```python
from build123d import *

# Parameters (mm, degrees)
F1_DEPTH  = 6
F3_R      = 2.5
F4_DEPTH  = 25
F5_W      = 22.1
F5_H      = 30
F6_DEPTH  = 25
F7_R      = 8
F7_R_2    = 12
F7_R_3    = 1.25
F8_DEPTH  = 25
F9_R      = 1
F10_DEPTH = 3
F11_R     = 1
F12_DEPTH = 3


with BuildPart() as f1:
    # F0 (on Top) → F1 (new body)
    with BuildSketch(Plane.XY):
        Polygon((0, -73.897189), (0, -125), (224, -125), (224, -73.897189), (383.758505, -30), (440.241495, -14.480047), (431.678371, 14.271873), (383.758505, 0), (224, 0), (224, 27.111), (0, 27.111), (0, 0), (-159.758505, 0), (-207.678371, 14.271873), (-216.241495, -14.480047), (-159.758505, -30), align=None)
    extrude(amount=F1_DEPTH)

    # F3 (on face) → F4 (cut)
    with BuildSketch(Plane(origin=(0, 0, 0), x_dir=(1, 0, 0), z_dir=(0, 0, -1))):
        with Locations((132, 60)):
            Circle(F3_R)
        with Locations((132, 20)):
            Circle(F3_R)
        with Locations((92, 60)):
            Circle(F3_R)
        with Locations((92, 20)):
            Circle(F3_R)
    extrude(amount=-F4_DEPTH, mode=Mode.SUBTRACT)

    # F5 (on face) → F6 (cut)
    with BuildSketch(Plane(origin=(0, 0, 0), x_dir=(1, 0, 0), z_dir=(0, 0, -1))):
        with Locations((192.95, 60)):
            Rectangle(F5_W, F5_H)
    extrude(amount=-F6_DEPTH, mode=Mode.SUBTRACT)

    # F7 (on face) → F8 (cut)
    with BuildSketch(Plane(origin=(0, 0, 0), x_dir=(1, 0, 0), z_dir=(0, 0, -1))):
        with BuildLine():
            Line((209.65, 22.101725), (209.65, 27.898275))
            ThreePointArc((209.65, 27.898275), (197.65, 25), (209.65, 22.101725))
        make_face()
        with Locations((182, 25)):
            Circle(F7_R)
        with Locations((30, 55)):
            Circle(F7_R_2)
        with Locations((20.5, 67)):
            Circle(F7_R_3)
        with Locations((39.5, 43)):
            Circle(F7_R_3)
    extrude(amount=-F8_DEPTH, mode=Mode.SUBTRACT)

    # F9 (on face) → F10 (join)
    with BuildSketch(Plane.XY.offset(6)):
        Polygon((430.556438, 4.025349), (425.764451, 2.598162), (427.191639, -2.193825), (431.983625, -0.766638), align=None)
        with Locations((428.874038, 0.915762)):
            Circle(F9_R, mode=Mode.SUBTRACT)
        Polygon((390.30375, -7.963025), (385.511763, -9.390212), (386.938951, -14.182199), (391.730937, -12.755011), align=None)
        with Locations((388.62135, -11.072612)):
            Circle(F9_R, mode=Mode.SUBTRACT)
    extrude(amount=F10_DEPTH)

    # F11 (on face) → F12 (join)
    with BuildSketch(Plane.XY.offset(6)):
        Polygon((-203.191639, -2.193825), (-201.764451, 2.598162), (-206.556438, 4.025349), (-207.983625, -0.766638), align=None)
        with Locations((-204.874038, 0.915762)):
            Circle(F11_R, mode=Mode.SUBTRACT)
        Polygon((-162.938951, -14.182199), (-161.511763, -9.390212), (-166.30375, -7.963025), (-167.730937, -12.755011), align=None)
        with Locations((-164.62135, -11.072612)):
            Circle(F11_R, mode=Mode.SUBTRACT)
    extrude(amount=F12_DEPTH)


solid = f1.part
```
Input: part model. Units: mm. Frame: model coordinates. A direction names the side the tool comes from. Coordinates: 2 decimals unless noted, no trailing zeros. Write each loop counter-clockwise with the first axis right and the second up, starting at its lowest first coordinate (ties: lowest second). Pieces come first, ordered by that corner, then holes.
1) Section B-B on y = -102.5. Output: boundary loops of the cut face in (x, z).
2) Section C-C on x = 342.5. Output: boundary loops of the cut face in (y, z), and give its area (3 significant figures).
3) Set-up query: faces 3 (the flat face through (-183.383, 7.036, 2.958)), 4 (the cylindrical face through (189.63, -27.4, 2.96)). Return all of +Z, -Z, +X, -X, +Y, -Y with unobstructed straight access to the full face (end or side cutting, diameter ignored); none if empty.
4) Mould query, pull axis X, two halves, no side actions, for faces 1 (the flat face through (408.054, 7.236, 2.958)), 2 (the flat face through (107, -31, 0)). Classes: pulls with the +X half, pulls with the -X half, needs draft (parallel to the pull), parting line crosses it, or undercut.
5) Section A-A on x = 30. Output: boundary loops of the cut face in (y, z), and give its area (3 significant figures).
6) Material intervals for line 1 along Y through (x, z) = (182, 2.95); line 2 along Y through (x, z) = (201, 4); line 3 along Y through (x, z) = (197.5, 3.5), sorted ascending.
7) Pin query (flat end, axial travel): pin 1 Ø1 at (x, y) = (-205, 1) entering from +Z; pin 2 Ø21.5 at (x, y) = (30, -55) entering from +Z; pin 3 Ø1.8 at (y, z) = (-102.5, 3.5) entering from -X; pin 4 Ø5 at (x, z) = (-44, 4) entering from +Y. Return the tip coordinate at first contact, or that it passes through.
Check result:
1. outline: (0, 0) - (224, 0) - (224, 6) - (0, 6) - close
2. outline: (-41.34, 0) - (0, 0) - (0, 6) - (-41.34, 6) - close
2. area: 248 mm2
3. face 3: +Z, -Z, +Y
3. face 4: +Z, -Z
4. face 1: undercut
4. face 2: needs draft
5. outline: (-125, 0) - (-67, 0) - (-67, 6) - (-125, 6) - close; (-43, 0) - (27.11, 0) - (27.11, 6) - (-43, 6) - close
5. area: 769 mm2
6. line 1: y = -125 to -75, -45 to -33, -17 to 27.11
6. line 2: y = -125 to -75, -45 to -30.6, -19.4 to 27.11
6. line 3: y = -125 to -75, -45 to 27.11
7. pin 1: stops at z = 6
7. pin 2: passes through
7. pin 3: stops at x = 0
7. pin 4: stops at y = 0
